Here's how the part is built. I have some questions about the finished solid (model axes, mm). Face numbers are marked on the shaded views. A direction names the side the tool comes from. Round coordinates to 2 decimals unless told otherwise and drop trailing zeros. Write each loop counter-clockwise with the first axis right and the second up, starting at its lowest first coordinate (ties: lowest second). Pieces come first, ordered by that corner, then holes. Notation, with made-up numbers: M 3.25,-1.5 L 17.25,-1.5 A23 ccw 17.25,9.5 Z; hole C 62.5,73.5 d7. An arc over 180 degrees is marked long. Write item = value, one per line. Start each with the question number.
(1) Will these pins go through, and if not, where does the flat tip stop? pin 1 Ø4 at (x, y) = (30.5, 60) entering from -Z; pin 2 Ø1.5 at (x, z) = (14, -7) entering from +Y; pin 3 Ø3 at (x, y) = (16, 52.5) entering from +Z; pin 4 Ø4 at (y, z) = (38, -38) entering from -X.
(2) I want a section at B-B (z = 0). List the corners of the cut face in (x, y) for me.
(3) On a 3-axis mill with a long thin cutter (end or side, diameter ignored), from which of +Z, -Z, +X, -X, +Y, -Y can I reach the whole of each face in a straight line? I mean the marked faces 1, 2, 3 and 4. Say none if no direction works.
(4) I want a section at C-C (y = 36.5). List the corners of the cut face in (x, z) for me, and give its area (3 significant figures).
(5) If we mould it in two halves opening along Z, with no side actions, what happens to the marked faces 5, 6, 7 and 8? For each: released by +Z, released by -Z, zero draft, split by the parting line, or undercut.
(6) I want a section at A-A (y = 12.5). List the corners of the cut face in (x, z) for me, and give its area (3 significant figures).
(7) I need wall thicknesses on line 1 along Y through (x, z) = (-14, 64.5); line 2 along Z through (x, y) = (-2, 45); line 3 along Y through (x, z) = (-13, 3). Which ranges of each line are inside material? Lowest first, please.
(8) I want a section at D-D (y = 72.5). List the corners of the cut face in (x, z) for me.
```python
from build123d import *

# Parameters (mm, degrees)
F2_R     = 7.5
F2_R_2   = 32
F3_DEPTH = 33


with BuildPart() as f1:
    # F0 (on Right) → F1 (revolve)
    with BuildSketch(Plane.YZ):
        with BuildLine():
            Line((3, 32), (3, 0))
            Line((3, 0), (21, 0))
            Line((21, 0), (21, 26))
            Line((21, 26), (63, 26))
            Line((63, 26), (63, 29))
            Line((63, 29), (93, 31))
            Line((93, 31), (93, 39))
            Line((93, 39), (85, 39))
            Line((85, 39), (85, 45))
            Line((85, 45), (55, 45))
            Line((55, 45), (55, 33.200345))
            ThreePointArc((55, 33.200345), (52.308743, 28.765291), (47.132118, 29.104585))
            Line((47.132118, 29.104585), (33, 39))
            Line((33, 39), (0, 39))
            Line((0, 39), (0, 32))
            Line((0, 32), (3, 32))
        make_face()
    revolve(axis=Axis((0, 12, 0), (0, 1, 0)))

    # F2 (on face) → F3 (join)
    with BuildSketch(Plane.XZ):
        with BuildLine():
            Line((36.607976, 13.448276), (17.834655, 64.551724))
            ThreePointArc((17.834655, 64.551724), (1.340517, 76.952652), (-16.734909, 66.996823))
            Line((-16.734909, 66.996823), (-36.563187, 13.569575))
            ThreePointArc((-36.563187, 13.569575), (0.064652, 38.999946), (36.607976, 13.448276))
        make_face()
        with BuildLine():
            ThreePointArc((0, 50.5), (-5.303301, 63.303301), (7.5, 58))
            ThreePointArc((7.5, 58), (5.303301, 52.696699), (0, 50.5))
        make_face(mode=Mode.SUBTRACT)
        with BuildLine():
            ThreePointArc((36.607976, -13.448276), (0.064652, -38.999946), (-36.563187, -13.569575))
            Line((-36.563187, -13.569575), (-16.734909, -66.996823))
            ThreePointArc((-16.734909, -66.996823), (1.340517, -76.952652), (17.834655, -64.551724))
            Line((17.834655, -64.551724), (36.607976, -13.448276))
        make_face()
        with Locations((0, -58)):
            Circle(F2_R, mode=Mode.SUBTRACT)
        with BuildLine():
            ThreePointArc((39, 0), (38.397337, 6.829676), (36.607976, 13.448276))
            ThreePointArc((36.607976, 13.448276), (0.064652, 38.999946), (-36.563187, 13.569575))
            ThreePointArc((-36.563187, 13.569575), (-39, 0), (-36.563187, -13.569575))
            ThreePointArc((-36.563187, -13.569575), (0.064652, -38.999946), (36.607976, -13.448276))
            ThreePointArc((36.607976, -13.448276), (38.397337, -6.829676), (39, 0))
        make_face()
        Circle(F2_R_2, mode=Mode.SUBTRACT)
    extrude(amount=-F3_DEPTH)


solid = f1.part
```
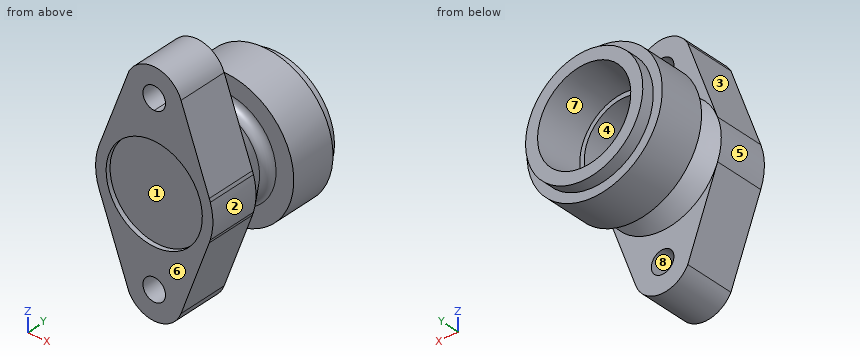
Returned:
q1.pin_1 = -34.82
q1.pin_2 = 21
q1.pin_3 = 25.79
q1.pin_4 = through
q2.outline = M -45,55 L -33.2,55 A5 cw -29.1,47.13 L -39,33 L -39,0 L -32,0 L -32,3 L 32,3 L 32,0 L 39,0 L 39,33 L 29.1,47.13 A5 cw 33.2,55 L 45,55 L 45,85 L 39,85 L 39,93 L 31,93 L 29,63 L 26,63 L 26,21 L -26,21 L -26,63 L -29,63 L -31,93 L -39,93 L -39,85 L -45,85 Z
q3.face_1 = -Y
q3.face_2 = +X, -Y
q3.face_3 = +Z, -X, -Y
q3.face_4 = +Y
q4.outline = C 0,0 d73.1; hole C 0,0 d52
q4.area = 2,070 mm²
q5.face_5 = split by the parting line
q5.face_6 = zero draft
q5.face_7 = undercut
q5.face_8 = undercut
q6.outline = M -36.56,-13.57 L -16.73,-67 A19 ccw 17.83,-64.55 L 36.61,-13.45 A39 ccw 37.3,-11.39 A39 ccw 37.3,11.39 A39 ccw 36.61,13.45 L 17.83,64.55 A19 ccw -16.73,67 L -36.56,13.57 A39 ccw Z; hole C 0,-58 d15; hole C 0,58 d15
q6.area = 7,900 mm²
q7.line_1 = 0 to 33
q7.line_2 = -30.53 to -25.92, 25.92 to 30.53
q7.line_3 = 3 to 21
q8.outline = C 0,0 d90; hole C 0,0 d59.27
